from build123d import *

# Parameters (mm, degrees)
BOX021003010009_W     = 10
BOX021003010009_H     = 10
BOX021003010009_DEPTH = 12
BOX021003010006_W     = 45
BOX021003010006_H     = 20
BOX021003010006_DEPTH = 30
BOX021003010005_W     = 20
BOX021003010005_H     = 90
BOX021003010005_DEPTH = 30


with BuildPart() as obj1:
    # Box021003010009 → Box021003010009 (new body)
    with BuildSketch(Plane(origin=(10, 125, 20), x_dir=(1, 0, 0), z_dir=(0, 0, 1))):
        with Locations((5, 5)):
            Rectangle(BOX021003010009_W, BOX021003010009_H)
    extrude(amount=BOX021003010009_DEPTH)


with BuildPart() as obj2:
    # Box021003010006 → Box021003010006 (new body)
    with BuildSketch(Plane(origin=(5, 185, 0), x_dir=(1, 0, 0), z_dir=(0, 0, 1))):
        with Locations((22.5, 10)):
            Rectangle(BOX021003010006_W, BOX021003010006_H)
    extrude(amount=BOX021003010006_DEPTH)


with BuildPart() as obj3:
    # Box021003010005 → Box021003010005 (new body)
    with BuildSketch(Plane(origin=(5, 115, 0), x_dir=(1, 0, 0), z_dir=(0, 0, 1))):
        with Locations((10, 45)):
            Rectangle(BOX021003010005_W, BOX021003010005_H)
    extrude(amount=BOX021003010005_DEPTH)

    # Fusion007: union obj2
    add(obj2.part)

    # Cut011: cut obj1
    add(obj1.part, mode=Mode.SUBTRACT)


solid = obj3.part
Input: part model. Units: mm. Frame: model coordinates. A direction names the side the tool comes from. Give positions to 0.01 mm unless a question says otherwise; leave off trailing zeros. Order: outer loops, then holes, each group sorted by start corner. A loop starts at its lowest first (then second) coordinate and runs counter-clockwise, first axis right, second up. Notation, with made-up numbers: (-28, 89) -> (-17, 89) arc R10 cw to (-17, 96) -> close; hole circle Ø2 at (19, 40). An arc over 180 degrees is marked (long way). Use one line per item in the form item = value.
1) Section A-A, the plane z = 22. Return loops of the section in (x, y).
Response values:
outline = (5, 115) -> (25, 115) -> (25, 185) -> (50, 185) -> (50, 205) -> (5, 205) -> close; hole (10, 125) -> (20, 125) -> (20, 135) -> (10, 135) -> close
2) Section D-D, the plane y = 158. Return loops of the section in (x, z), and give its area (3 significant figures).
Response values:
outline = (5, 0) -> (25, 0) -> (25, 30) -> (5, 30) -> close
area = 600 mm^2
3) Section B-B, the plane x = 16.5. Return loops of the section in (y, z).
Response values:
outline = (115, 0) -> (205, 0) -> (205, 30) -> (135, 30) -> (135, 20) -> (125, 20) -> (125, 30) -> (115, 30) -> close
4) Section C-C, the plane z = 6.75. Return loops of the section in (x, y), and give its area (3 significant figures).
Response values:
outline = (5, 115) -> (25, 115) -> (25, 185) -> (50, 185) -> (50, 205) -> (5, 205) -> close
area = 2,300 mm^2
5) Mould query, pull axis X, two halves, no side actions, for faces 1 (the flat face through (50, 195, 15)), 2 (the flat face through (37, 185, 15)), 3 (the flat face through (15, 130, 20)). Classes: pulls with the +X half, pulls with the -X half, needs draft (parallel to the pull), parting line crosses it, or undercut.
Response values:
face_1 = pulls with the +X half
face_2 = needs draft
face_3 = undercut
6) First-contact query: pin 1 Ø10 at (x, z) = (35.5, 20) entering from -Y; pin 2 Ø6 at (y, z) = (170, 20.5) entering from +X; pin 3 Ø4 at (x, y) = (28.5, 155.5) entering from -Z; pin 4 Ø1.5 at (x, y) = (24.5, 139) entering from -Z. Flat tips, straight axial feed; report the tip coordinate or a pass-through.
Response values:
pin_1 = 185
pin_2 = 25
pin_3 = through
pin_4 = 0
7) Line query: probe 1 along X at (y, z) = (130.5, 24); probe 2 along X at (y, z) = (157.5, 15.25); probe 3 along Y at (x, z) = (41, 6.75). Output: solid intervals per line, ascending.
Response values:
probe_1 = 5 to 10, 20 to 25
probe_2 = 5 to 25
probe_3 = 185 to 205
8) Reachability of faces 4 (the flat face through (20, 130, 25)), 5 (the flat face through (27, 205, 15)), 6 (the flat face through (25, 150, 15)) from +Z, -Z, +X, -X, +Y, -Y: full face, straight path, thin tool, end or side. Return the list, or none.
Response values:
face_4 = +Z
face_5 = +Z, -Z, +X, -X, +Y
face_6 = +Z, -Z, +X, -Y
